Read the model definition and answer for the solid it produces. Units are mm, in the model's axes. Face numbers are marked on the shaded views. A direction names the side the tool comes from. Coordinates: 2 decimals unless noted, no trailing zeros. Loops run counter-clockwise (first coordinate to the right, second up) from the corner with the lowest first, then second, coordinate; pieces in that order, holes last. Notation, with made-up numbers: M 89.25,56 L 143.25,56 A26 cw 143.25,87 Z; hole C 45,29.25 d1. An arc over 180 degrees is marked long. Put each result on its own line as item: value.
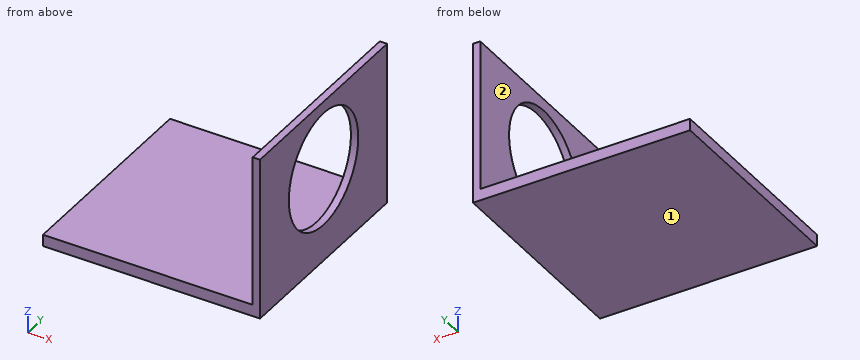
from build123d import *

# Parameters (mm, degrees)
F0_W     = 457.2
F0_H     = 457.2
F1_DEPTH = 25.4
F2_W     = 457.2
F2_H     = 355.6
F3_DEPTH = 15.875
F4_R     = 124.99975
F5_DEPTH = 15.875


with BuildPart() as f1:
    # F0 (on Top) → F1 (new body)
    with BuildSketch(Plane.XY):
        Rectangle(F0_W, F0_H)
    extrude(amount=F1_DEPTH)

    # F2 (on face) → F3 (join)
    with BuildSketch(Plane.YZ.offset(228.6)):
        with Locations((0, 177.8)):
            Rectangle(F2_W, F2_H)
    extrude(amount=F3_DEPTH)

    # F4 (on face) → F5 (cut, through all)
    with BuildSketch(Plane.YZ.offset(244.475)):
        with Locations((0, 205.20025)):
            Circle(F4_R)
    extrude(amount=-F5_DEPTH, mode=Mode.SUBTRACT)


solid = f1.part
1) Straight lines are drawn through the part: line 1 (Z direction, x = 234, y = 0); line 2 (X direction, y = -182, z = 134) (3 decimals); line 3 (Z direction, x = -47.5, y = 128). For each, find the intervals that lie inside material, in ascending order. Write a range as [from, to].
Answer list:
line 1: z = [0, 80.2], [330.2, 355.6]
line 2: x = [228.6, 244.475]
line 3: z = [0, 25.4]
2) Which of the six approach directions +Z, -Z, +X, -X, +Y, -Y give full straight-line access (tool end or side, diameter ignored) to the marked faces 1 and 2?
Answer list:
face 1: -Z, +X, -X, +Y, -Y
face 2: +Z, -X, +Y, -Y
3) Find section B-B, the plane z = 260.5. Write down the section's boundary in (x, y) (3 decimals).
Answer list:
outline: M 228.6,-228.6 L 244.475,-228.6 L 244.475,-112.102 L 228.6,-112.102 Z; M 228.6,112.102 L 244.475,112.102 L 244.475,228.6 L 228.6,228.6 Z
4) Find section D-D, the plane z = 182.5. Write down the section's boundary in (x, y) (3 decimals).
Answer list:
outline: M 228.6,-228.6 L 244.475,-228.6 L 244.475,-122.921 L 228.6,-122.921 Z; M 228.6,122.921 L 244.475,122.921 L 244.475,228.6 L 228.6,228.6 Z
5) Find section C-C, the plane y = -90.5. Write down the section's boundary in (x, z) (3 decimals), plus the area to 3 significant figures.
Answer list:
outline: M -228.6,0 L 244.475,0 L 244.475,118.976 L 228.6,118.976 L 228.6,25.4 L -228.6,25.4 Z; M 228.6,291.425 L 244.475,291.425 L 244.475,355.6 L 228.6,355.6 Z
area: 14,500 mm^2
6) Given pin 1 Ø4 at (x, y) = (-68.5, -179) entering from +Z; pin 2 Ø1 at (y, z) = (166, 162) entering from -X, each flat-ended and moving along its own axis, determine where each tip first touches the part or whether it passes through.
Answer list:
pin 1: stops at z = 25.4
pin 2: stops at x = 228.6
7) Find section A-A, the plane y = 0. Write down the section's boundary in (x, z) (1 decimal).
Answer list:
outline: M -228.6,0 L 244.5,0 L 244.5,80.2 L 228.6,80.2 L 228.6,25.4 L -228.6,25.4 Z; M 228.6,330.2 L 244.5,330.2 L 244.5,355.6 L 228.6,355.6 Z
